```python
from build123d import *

# Parameters (mm, degrees)
F1_DEPTH  = 2.159
F3_DEPTH  = 2.413
F5_DEPTH  = 2.413
F7_DEPTH  = 2.413
F9_DEPTH  = 2.413
F11_DEPTH = 6.35
F14_R     = 7.5311
F15_DEPTH = 6.35
F16_R     = 5.08
F17_R     = 1.905
F18_DEPTH = 18.162


with BuildPart() as f1:
    # F0 (on Top) → F1 (new body)
    with BuildSketch(Plane.XY):
        with BuildLine():
            Line((18.288, 20.2184), (2.54, 20.2184))
            ThreePointArc((2.54, 20.2184), (0.743949, 19.474451), (0, 17.6784))
            Line((0, 17.6784), (0, 2.54))
            ThreePointArc((0, 2.54), (0.743949, 0.743949), (2.54, 0))
            Line((2.54, 0), (18.288, 0))
            ThreePointArc((18.288, 0), (20.084051, 0.743949), (20.828, 2.54))
            Line((20.828, 2.54), (20.828, 17.6784))
            ThreePointArc((20.828, 17.6784), (20.084051, 19.474451), (18.288, 20.2184))
        make_face()
    extrude(amount=F1_DEPTH)

    # F2 (on face) → F3 (join)
    with BuildSketch(Plane.XY.offset(2.159)):
        with BuildLine():
            Line((20.955, 22.8092), (-0.127, 22.8092))
            ThreePointArc((-0.127, 22.8092), (-1.923051, 22.065251), (-2.667, 20.2692))
            Line((-2.667, 20.2692), (-2.667, -0.0508))
            ThreePointArc((-2.667, -0.0508), (-1.923051, -1.846851), (-0.127, -2.5908))
            Line((-0.127, -2.5908), (20.955, -2.5908))
            ThreePointArc((20.955, -2.5908), (22.751051, -1.846851), (23.495, -0.0508))
            Line((23.495, -0.0508), (23.495, 20.2692))
            ThreePointArc((23.495, 20.2692), (22.751051, 22.065251), (20.955, 22.8092))
        make_face()
    extrude(amount=F3_DEPTH)



with BuildPart() as f5:
    # F4 (on face) → F5 (new body)
    with BuildSketch(Plane.XY.offset(9.398)):
        with BuildLine():
            ThreePointArc((0, 2.54), (0.743949, 0.743949), (2.54, 0))
            Line((2.54, 0), (18.288, 0))
            ThreePointArc((18.288, 0), (20.084051, 0.743949), (20.828, 2.54))
            Line((20.828, 2.54), (20.828, 17.6784))
            ThreePointArc((20.828, 17.6784), (20.084051, 19.474451), (18.288, 20.2184))
            Line((18.288, 20.2184), (2.54, 20.2184))
            ThreePointArc((2.54, 20.2184), (0.743949, 19.474451), (0, 17.6784))
            Line((0, 17.6784), (0, 2.54))
        make_face()
    extrude(amount=F5_DEPTH)

    # F6 (on face) → F7 (join)
    with BuildSketch(Plane.XY.offset(6.985)):
        with BuildLine():
            Line((-2.667, 20.2692), (-2.667, -0.0508))
            ThreePointArc((-2.667, -0.0508), (-1.923051, -1.846851), (-0.127, -2.5908))
            Line((-0.127, -2.5908), (20.955, -2.5908))
            ThreePointArc((20.955, -2.5908), (22.751051, -1.846851), (23.495, -0.0508))
            Line((23.495, -0.0508), (23.495, 20.2692))
            ThreePointArc((23.495, 20.2692), (22.751051, 22.065251), (20.955, 22.8092))
            Line((20.955, 22.8092), (-0.127, 22.8092))
            ThreePointArc((-0.127, 22.8092), (-1.923051, 22.065251), (-2.667, 20.2692))
        make_face()
    extrude(amount=F7_DEPTH)


with BuildPart() as f1_1:
    add(f1.part)

    add(f5.part)  # F9 merges F5
    # F8 (on face) → F9 (join)
    with BuildSketch(Plane.XY.offset(4.572)):
        with BuildLine():
            ThreePointArc((0, 2.54), (0.743949, 0.743949), (2.54, 0))
            Line((2.54, 0), (18.288, 0))
            ThreePointArc((18.288, 0), (20.084051, 0.743949), (20.828, 2.54))
            Line((20.828, 2.54), (20.828, 17.6784))
            ThreePointArc((20.828, 17.6784), (20.084051, 19.474451), (18.288, 20.2184))
            Line((18.288, 20.2184), (2.54, 20.2184))
            ThreePointArc((2.54, 20.2184), (0.743949, 19.474451), (0, 17.6784))
            Line((0, 17.6784), (0, 2.54))
        make_face()
    extrude(amount=F9_DEPTH)

    # F10 (on face) → F11 (join)
    with BuildSketch(Plane.XY.offset(11.811)):
        with BuildLine():
            Line((20.955, 22.8092), (-0.127, 22.8092))
            ThreePointArc((-0.127, 22.8092), (-1.923051, 22.065251), (-2.667, 20.2692))
            Line((-2.667, 20.2692), (-2.667, -0.0508))
            ThreePointArc((-2.667, -0.0508), (-1.923051, -1.846851), (-0.127, -2.5908))
            Line((-0.127, -2.5908), (20.955, -2.5908))
            ThreePointArc((20.955, -2.5908), (22.751051, -1.846851), (23.495, -0.0508))
            Line((23.495, -0.0508), (23.495, 20.2692))
            ThreePointArc((23.495, 20.2692), (22.751051, 22.065251), (20.955, 22.8092))
        make_face()
    extrude(amount=F11_DEPTH)

    # F14 (on face) → F15 (cut)
    with BuildSketch(Plane(origin=(0, 0, 0), x_dir=(1, 0, 0), z_dir=(0, 0, -1))):
        with Locations((10.414, -10.1092)):
            Circle(F14_R)
    extrude(amount=-F15_DEPTH, mode=Mode.SUBTRACT)

    # F16
    f16_edges = [f1_1.edges().sort_by_distance(p)[0] for p in [
        (2.8829, 10.1092, 6.35),
    ]]
    fillet(f16_edges, radius=F16_R)

    # F17 (on face) → F18 (cut, through all)
    with BuildSketch(Plane.XY.offset(18.161)):
        with Locations((10.414, 10.1092)):
            Circle(F17_R)
    extrude(amount=-F18_DEPTH, mode=Mode.SUBTRACT)


solid = f1_1.part
```
Can you work these out from the model? Positions are in its coordinate system, mm. A direction names the side the tool comes from. Coordinates: 2 decimals unless noted, no trailing zeros. Loops run counter-clockwise (first coordinate to the right, second up) from the corner with the lowest first, then second, coordinate; pieces in that order, holes last. Notation, with made-up numbers: (-15, -20) -> (-5, -20) arc R19 cw to (-5, -8) -> close; hole circle Ø9 at (15.5, 30.5). An arc over 180 degrees is marked (long way). Put each result on its own line as item: value. Start each with the question number.
Q1. I want a section at A-A (z = 11). Write out the boundary of the cut face in (x, y) (3 decimals), plus the area to 3 significant figures.
Q2. If I drill on line 1 (Z direction, x = 0.75, y = -1) (3 decimals); line 2 (X direction, y = 12.75, z = 11.5); line 3 (Y direction, x = 12.25, z = 2.5), over which ranges is the centre line in solid material (lowest first)? Write a range as [from, to].
Q3. Thinking about a two-plate mould opening in Z: for faces 6 (the face through (10, -2.591, 15)), 7 (the face through (10, 7, 18.161)), 8 (the face through (20.104, 19.455, 5.762)), which applies, pulls with the +Z half, pulls with the -Z half, needs draft (parallel to the pull), parting line crosses it, or undercut?
Q4. I'm going to push flat-ended pins straight in: P1, Ø5, axis at x = 10.41, y = 10.11, coming from the -Z side; P2, Ø1.2, axis at y = 11.5, z = 5.5, coming from the -X side; P3, Ø1.5, axis at x = 10.5, y = 9, coming from the -Z side; P4, Ø1.1, axis at x = 13.5, z = 0.5, coming from the -Y side. Where does each tip first touch, or does it pass through?
Q5. For faces 1 (the face through (17.6, 7.85, 0.63)), 2 (the face through (20.06, 0.72, 5.76)), 3 (the face through (10, 0, 1)), 4 (the face through (0.724, 0.764, 10.588)), 5 (the face through (11, 20.218, 6)), which set-ups out of +Z, -Z, +X, -X, +Y, -Y let a thin tool reach every point of the face, with its end or its side?
Q6. I want a section at B-B (x = 18.75). Write out the boundary of the cut face in (y, z) (3 decimals), plus the area to 3 significant figures.
Q7. I want a section at C-C (y = 1.5). Write out the boundary of the cut face in (x, z) (3 decimals), plus the area to 3 significant figures.
Taken from the geometry:
1. outline: (0, 2.54) arc R2.54 ccw to (2.54, 0) -> (18.288, 0) arc R2.54 ccw to (20.828, 2.54) -> (20.828, 17.678) arc R2.54 ccw to (18.288, 20.218) -> (2.54, 20.218) arc R2.54 ccw to (0, 17.678) -> close; hole circle Ø3.81 at (10.414, 10.109)
1. area: 404 mm2
2. line 1: z = [2.159, 4.572], [6.985, 9.398], [11.811, 18.161]
2. line 2: x = [0, 20.83]
2. line 3: y = [-2.59, 2.96], [17.26, 22.81]
3. face 6: needs draft
3. face 7: pulls with the +Z half
3. face 8: undercut
4. P1: stops at z = 6.35
4. P2: stops at x = 0
4. P3: passes through
4. P4: stops at y = 0
5. face 1: -Z
5. face 2: +X, -Y
5. face 3: -Z, +X, -X, -Y
5. face 4: -X, -Y
5. face 5: +X, -X, +Y
6. outline: (-2.591, 2.159) -> (0.042, 2.159) -> (0.042, 0) -> (20.176, 0) -> (20.176, 2.159) -> (22.809, 2.159) -> (22.809, 4.572) -> (20.176, 4.572) -> (20.176, 6.985) -> (22.809, 6.985) -> (22.809, 9.398) -> (20.176, 9.398) -> (20.176, 11.811) -> (22.809, 11.811) -> (22.809, 18.161) -> (-2.591, 18.161) -> (-2.591, 11.811) -> (0.042, 11.811) -> (0.042, 9.398) -> (-2.591, 9.398) -> (-2.591, 6.985) -> (0.042, 6.985) -> (0.042, 4.572) -> (-2.591, 4.572) -> close
6. area: 425 mm2
7. outline: (-2.667, 2.159) -> (0.223, 2.159) -> (0.223, 0) -> (20.605, 0) -> (20.605, 2.159) -> (23.495, 2.159) -> (23.495, 4.572) -> (20.605, 4.572) -> (20.605, 6.985) -> (23.495, 6.985) -> (23.495, 9.398) -> (20.605, 9.398) -> (20.605, 11.811) -> (23.495, 11.811) -> (23.495, 18.161) -> (-2.667, 18.161) -> (-2.667, 11.811) -> (0.223, 11.811) -> (0.223, 9.398) -> (-2.667, 9.398) -> (-2.667, 6.985) -> (0.223, 6.985) -> (0.223, 4.572) -> (-2.667, 4.572) -> close
7. area: 435 mm2
